from build123d import *

# Parameters (mm, degrees)
F1_DEPTH = 12
F2_R     = 1.75
F3_DEPTH = 12
F4_DEPTH = 4


with BuildPart() as f1:
    # F0 (on Top) → F1 (new body)
    with BuildSketch(Plane.XY):
        with BuildLine():
            Line((0, 12), (0, 0))
            Line((0, 0), (22.062746, 0))
            ThreePointArc((22.062746, 0), (30, 7), (37.937254, 0))
            Line((37.937254, 0), (48, 0))
            Line((48, 0), (48, 12))
            Line((48, 12), (0, 12))
        make_face()
    extrude(amount=F1_DEPTH)

    # F2 (on face) → F3 (cut, through all)
    with BuildSketch(Plane(origin=(0, 12, 0), x_dir=(-1, 0, 0), z_dir=(0, 1, 0))):
        with Locations((-42, 6)):
            Circle(F2_R)
        with Locations((-16, 6)):
            Circle(F2_R)
    extrude(amount=-F3_DEPTH, mode=Mode.SUBTRACT)

    # F2 (on face) → F4 (cut)
    with BuildSketch(Plane(origin=(0, 12, 0), x_dir=(-1, 0, 0), z_dir=(0, 1, 0))):
        Polygon((-39, 4.267949), (-39, 7.732051), (-42, 9.464102), (-45, 7.732051), (-45, 4.267949), (-42, 2.535898), align=None)
        with Locations((-42, 6)):
            Circle(F2_R, mode=Mode.SUBTRACT)
        Polygon((-13, 7.732051), (-16, 9.464102), (-19, 7.732051), (-19, 4.267949), (-16, 2.535898), (-13, 4.267949), align=None)
        with Locations((-16, 6)):
            Circle(F2_R, mode=Mode.SUBTRACT)
    extrude(amount=-F4_DEPTH, mode=Mode.SUBTRACT)


solid = f1.part
Part model, mm, in its own coordinate system. A direction names the side the tool comes from. Coordinates: 2 decimals unless noted, no trailing zeros. Loops run counter-clockwise (first coordinate to the right, second up) from the corner with the lowest first, then second, coordinate; pieces in that order, holes last. Notation, with made-up numbers: (-13.5, 86) - (16.5, 86) arc R25 ccw to (16.5, 125) - close; hole circle Ø10 at (58.25, 80). An arc over 180 degrees is marked (long way). Write each question's results on one line, items separated by ' | '. Start each with the question number.
Q1. Slice it at A-A on y = 2.75. Give the cut face in (x, z), and give its area (3 significant figures).
Q2. Slice it at C-C on y = 11. Give the cut face in (x, z).
Q3. Which spindle directions (+Z, -Z, +X, -X, +Y, -Y) get a long thin tool onto all of the face, cutting with end or side? Do faces 4 (the cylindrical face through (30, 7, 6)), 5 (the flat face through (19, 10, 6)). Say none if no direction does.
Q4. Slice it at B-B on z = 6. Give the cut face in (x, y).
Q5. Slice it at D-D on z = 11.25. Give the cut face in (x, y).
Q6. Two-plate mould, pull along Z, no slides. Class faces 1 (the flat face through (24, 6, 12)), 2 (the cylindrical face through (40.383, 4.056, 5.33)), 3 (the flat face through (44, 0, 6)): +Z half, -Z half, draft (parallel to the pull), parting line (faces both ways), or undercut.
Q7. Probe line 1 along Z through (x, y) = (42, 3); line 2 along X through (y, z) = (7.25, 4.5); line 3 along X through (y, z) = (4.75, 7.25). List the from-to ranges inside material, lowest first.
Answer:
1) outline: (0, 0) - (22.93, 0) - (22.93, 12) - (0, 12) - close; (37.07, 0) - (48, 0) - (48, 12) - (37.07, 12) - close; hole circle Ø3.5 at (16, 6); hole circle Ø3.5 at (42, 6) | area: 387 mm2
2) outline: (0, 0) - (48, 0) - (48, 12) - (0, 12) - close; hole (13, 4.27) - (16, 2.54) - (19, 4.27) - (19, 7.73) - (16, 9.46) - (13, 7.73) - close; hole (39, 4.27) - (42, 2.54) - (45, 4.27) - (45, 7.73) - (42, 9.46) - (39, 7.73) - close
3) face 4: +Z, -Z, -Y | face 5: +Y
4) outline: (0, 0) - (14.25, 0) - (14.25, 8) - (13, 8) - (13, 12) - (0, 12) - close; (17.75, 0) - (22.06, 0) arc R8 cw to (37.94, 0) - (40.25, 0) - (40.25, 8) - (39, 8) - (39, 12) - (19, 12) - (19, 8) - (17.75, 8) - close; (43.75, 0) - (48, 0) - (48, 12) - (45, 12) - (45, 8) - (43.75, 8) - close
5) outline: (0, 0) - (22.06, 0) arc R8 cw to (37.94, 0) - (48, 0) - (48, 12) - (0, 12) - close
6) face 1: +Z half | face 2: undercut | face 3: draft
7) line 1: z = 0 to 4.25, 7.75 to 12 | line 2: x = 0 to 15.1, 16.9 to 41.1, 42.9 to 48 | line 3: x = 0 to 14.78, 17.22 to 24.44, 35.56 to 40.78, 43.22 to 48
